Could you check a few things on this model? Use its own coordinates, in mm. A direction names the side the tool comes from. Round coordinates to 2 decimals unless told otherwise and drop trailing zeros. Write each loop counter-clockwise with the first axis right and the second up, starting at its lowest first coordinate (ties: lowest second). Pieces come first, ordered by that corner, then holes. Notation, with made-up numbers: M 11.5,40 L 57.5,40 A23 ccw 57.5,75 Z; hole C 17.5,4 d7. An arc over 180 degrees is marked long. One line per item, written item: value. Start each with the question number.
(1) Which directions (+Z, -Z, +X, -X, +Y, -Y) give clear straight access to the entire face, cutting with the end or side of a thin tool? Please do faces 4 (the face through (0, 86, 4)), 5 (the face through (1, 57, 8)), 6 (the face through (35, 93, 4)).
(2) I want a section at A-A on x = -37. Please give me the cut outline in (y, z).
(3) I'm going to push flat-ended pins straight in: pin 1 Ø3 at (y, z) = (110.5, 5) entering from -X; pin 2 Ø3 at (x, z) = (-33.5, 5.5) entering from +Y. Where does each tip first touch, or does it pass through?
(4) Thinking about a two-plate mould opening in X: for faces 1 (the face through (5, 91.82, 4)), 2 (the face through (29.93, 150.205, 3.944)), 3 (the face through (-35, 93, 4)), which applies, released by +X, released by -X, zero draft, split by the parting line, or undercut?
(5) If I drill on L1, parallel to Y at x = 21, z = 5.25; L2, parallel to Y at x = 15.5, z = 4.5; L3, parallel to Y at x = -37, z = 6, over which ranges is the centre line in solid material (lowest first)?
(6) I want a section at D-D on z = 3.5. Count the separate pieces of the cut face and the enclosed holes in it, and give its area (3 significant figures).
(7) I want a section at B-B on x = -15.5. Please give me the cut outline in (y, z), and give its area (3 significant figures).
(8) I want a section at C-C on y = 75. Please give me the cut outline in (x, z).
```python
from build123d import *

# Parameters (mm, degrees)
SKETCH2_R           = 4
SKETCH2_R_2         = 10
SKETCH2_R_3         = 2.5
SKETCH2_R_4         = 3.9
SKETCH2_W           = 10
SKETCH2_H           = 5
BOSS_EXTRUDE2_DEPTH = 8
SKETCH3_R           = 1.9
CUT_EXTRUDE1_DEPTH  = 10
CHAMFER1_SIZE       = 10


with BuildPart() as part:
    # Sketch2 → Boss-Extrude2 (new body)
    with BuildSketch(Plane.XY):
        with BuildLine():
            Line((50, -44.865381447), (-50, -44.865381447))
            Line((-50, -44.865381447), (-50, 25.134618553))
            Line((-50, 25.134618553), (-50, 40.864537659))
            ThreePointArc((-50, 40.864537659), (-49.414213562, 42.278751221), (-48, 42.864537659))
            Line((-48, 42.864537659), (-35, 42.864537659))
            Line((-35, 42.864537659), (-35, 155.134618553))
            Line((-35, 155.134618553), (35, 155.134618553))
            Line((35, 155.134618553), (35, 39.08785688))
            Line((35, 39.08785688), (50, 25.134618553))
            Line((50, 25.134618553), (50, -44.865381447))
        make_face()
        with Locations((-37, 15.134618553)):
            Circle(SKETCH2_R, mode=Mode.SUBTRACT)
        with Locations(Location((37, 15.134618553, 0), (0, 0, 180))):
            Circle(SKETCH2_R, mode=Mode.SUBTRACT)
        with Locations((0, 30.134618553)):
            Circle(SKETCH2_R_2, mode=Mode.SUBTRACT)
        with Locations((42, -39.865381447)):
            Circle(SKETCH2_R_3, mode=Mode.SUBTRACT)
        with Locations((21, -39.865381447)):
            Circle(SKETCH2_R_3, mode=Mode.SUBTRACT)
        with Locations((-43.787591992, 36.827877872)):
            Circle(SKETCH2_R, mode=Mode.SUBTRACT)
        with Locations((42, -11.865381447)):
            Circle(SKETCH2_R_3, mode=Mode.SUBTRACT)
        with Locations((21, -11.865381447)):
            Circle(SKETCH2_R_3, mode=Mode.SUBTRACT)
        with Locations(Location((-21, -11.865381447, 0), (0, 0, 180))):
            Circle(SKETCH2_R_3, mode=Mode.SUBTRACT)
        with Locations(Location((-42, -11.865381447, 0), (0, 0, 180))):
            Circle(SKETCH2_R_3, mode=Mode.SUBTRACT)
        with Locations(Location((-21, -39.865381447, 0), (0, 0, 180))):
            Circle(SKETCH2_R_3, mode=Mode.SUBTRACT)
        with Locations(Location((-42, -39.865381447, 0), (0, 0, 180))):
            Circle(SKETCH2_R_3, mode=Mode.SUBTRACT)
        with Locations((-16.01970462, 60.134618553)):
            Circle(SKETCH2_R_4, mode=Mode.SUBTRACT)
        with Locations((16.019778849, 60.134618553)):
            Circle(SKETCH2_R_4, mode=Mode.SUBTRACT)
        with Locations((-16.01970462, 137.048261945)):
            Circle(SKETCH2_R_4, mode=Mode.SUBTRACT)
        with Locations((16.019778849, 137.048261945)):
            Circle(SKETCH2_R_4, mode=Mode.SUBTRACT)
        with Locations((5, 86.183799898)):
            Rectangle(SKETCH2_W, SKETCH2_H, mode=Mode.SUBTRACT)
        with Locations((5, 94.319599175)):
            Rectangle(SKETCH2_W, SKETCH2_H, mode=Mode.SUBTRACT)
    extrude(amount=BOSS_EXTRUDE2_DEPTH)

    # Sketch3 → Cut-Extrude1 (cut)
    with BuildSketch(Plane.XY.offset(8)):
        with Locations((-15.5, 14.634618553)):
            Circle(SKETCH3_R)
        with Locations((-15.5, 45.634618553)):
            Circle(SKETCH3_R)
        with Locations((15.5, 45.634618553)):
            Circle(SKETCH3_R)
        with Locations((15.5, 14.634618553)):
            Circle(SKETCH3_R)
    extrude(amount=-CUT_EXTRUDE1_DEPTH, mode=Mode.SUBTRACT)

    # Chamfer1
    chamfer1_edges = [part.edges().sort_by_distance(p)[0] for p in [
        (-35, 155.134618553, 4),
        (35, 155.134618553, 4),
    ]]
    chamfer(chamfer1_edges, length=CHAMFER1_SIZE)


solid = part.part
```
Found:
1. face 4: +Z, -Z
1. face 5: +Z, +X, -X, +Y, -Y
1. face 6: +Z, -Z, +X, +Y
2. outline: M -44.87,0 L 11.13,0 L 11.13,8 L -44.87,8 Z; M 19.13,0 L 42.86,0 L 42.86,8 L 19.13,8 Z
3. pin 1: stops at x = -35
3. pin 2: stops at y = 148.13
4. face 1: undercut
4. face 2: released by +X
4. face 3: released by -X
5. L1: y = -44.87 to -42.37, -37.37 to -14.37, -9.37 to 155.13
5. L2: y = -44.87 to 12.73, 16.53 to 43.73, 47.53 to 56.27, 64 to 133.18, 140.91 to 155.13
5. L3: y = -44.87 to 11.13, 19.13 to 42.86
6. separate pieces: 1
6. enclosed holes: 22
6. area: 15,400 mm²
7. outline: M -44.87,0 L 12.73,0 L 12.73,8 L -44.87,8 Z; M 16.53,0 L 43.73,0 L 43.73,8 L 16.53,8 Z; M 47.53,0 L 56.27,0 L 56.27,8 L 47.53,8 Z; M 64,0 L 133.18,0 L 133.18,8 L 64,8 Z; M 140.91,0 L 155.13,0 L 155.13,8 L 140.91,8 Z
7. area: 1,420 mm²
8. outline: M -35,0 L 35,0 L 35,8 L -35,8 Z
